Part model, mm, in its own coordinate system. Face numbers are marked on the shaded views. A direction names the side the tool comes from. Coordinates: 2 decimals unless noted, no trailing zeros. Loops run counter-clockwise (first coordinate to the right, second up) from the corner with the lowest first, then second, coordinate; pieces in that order, holes last. Notation, with made-up numbers: (87, 27.25) -> (114, 27.25) arc R22 ccw to (114, 38.25) -> close; hole circle Ø7 at (-8.5, 3). An arc over 180 degrees is marked (long way). Use one line per item in the form item = value. Start each with the question number.
(1) Band-saw the part on C-C on y = 3. Give the cut face in (x, z).
(2) Drill centre lines: L1, parallel to X at y = 0, z = 21; L2, parallel to Y at x = 4.5, z = 21.75; L3, parallel to Z at x = 0, y = -1.75. Where is each one in solid material? Low to high. Write a range as [from, to].
(3) Pin check, flat tips, straight feed: P1, Ø1.8, axis at x = -4.5, y = 0, coming from the +Z side; P2, Ø5, axis at x = 1.5, y = 1, coming from the -Z side; P3, Ø1.3, axis at x = -4.5, y = -3.5, coming from the -Z side; P4, Ø1.8, axis at x = -0.5, z = 27, coming from the +Y side. Stop position of each tip, or through.
(4) Band-saw the part on B-B on z = 4.5. Give the cut face in (x, y), then the cut area to 3 significant figures.
(5) 3-axis set-ups, long thin cutter, end or side, ignore diameter. For the marked faces 1, 2, 3, 4 and 5: which of +Z, -Z, +X, -X, +Y, -Y reach the whole face in a straight line?
(6) Band-saw the part on A-A on z = 23. Give the cut face in (x, y), then the cut area to 3 significant figures.
(7) Band-saw the part on D-D on z = 29.5. Give the cut face in (x, y).
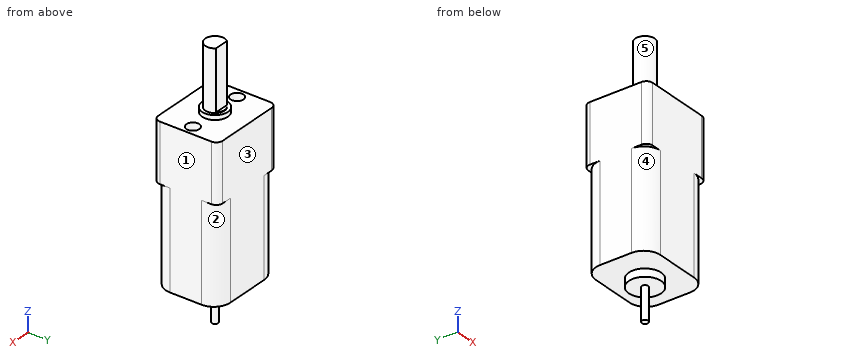
```python
from build123d import *

# Parameters (mm, degrees)
BOSS_EXTRUDE1_DEPTH        = 15
BOSS_EXTRUDE2_DEPTH        = 9
SKETCH3_R                  = 2
BOSS_EXTRUDE3_DEPTH        = 0.7
SKETCH4_R                  = 1.5
BOSS_EXTRUDE4_DEPTH        = 9.3
SKETCH5_W                  = 3
SKETCH5_H                  = 1
CUT_EXTRUDE1_DEPTH         = 9.2
SKETCH6_R                  = 2.5
BOSS_EXTRUDE5_DEPTH        = 1.2
SKETCH7_R                  = 0.5
BOSS_EXTRUDE6_DEPTH        = 5
M1_6_CLEARANCE_HOLE1_D     = 2
M1_6_CLEARANCE_HOLE1_DEPTH = 7
M1_6_CLEARANCE_HOLE1_TIP   = 0.600860619


with BuildPart() as part:
    # Sketch1 → Boss-Extrude1 (new body)
    with BuildSketch(Plane.XY):
        with BuildLine():
            Line((3.45, -5), (-3.45, -5))
            ThreePointArc((-3.45, -5), (-5.253122292, -4.253122292), (-6, -2.45))
            Line((-6, -2.45), (-6, 2.45))
            ThreePointArc((-6, 2.45), (-5.253122292, 4.253122292), (-3.45, 5))
            Line((-3.45, 5), (3.45, 5))
            ThreePointArc((3.45, 5), (5.253122292, 4.253122292), (6, 2.45))
            Line((6, 2.45), (6, -2.45))
            ThreePointArc((6, -2.45), (5.253122292, -4.253122292), (3.45, -5))
        make_face()
    extrude(amount=BOSS_EXTRUDE1_DEPTH)

    # Sketch2 → Boss-Extrude2 (add)
    with BuildSketch(Plane.XY.offset(15)):
        with BuildLine():
            Line((5, -5), (-5, -5))
            ThreePointArc((-5, -5), (-5.707106781, -4.707106781), (-6, -4))
            Line((-6, -4), (-6, 4))
            ThreePointArc((-6, 4), (-5.707106781, 4.707106781), (-5, 5))
            Line((-5, 5), (5, 5))
            ThreePointArc((5, 5), (5.707106781, 4.707106781), (6, 4))
            Line((6, 4), (6, -4))
            ThreePointArc((6, -4), (5.707106781, -4.707106781), (5, -5))
        make_face()
    extrude(amount=BOSS_EXTRUDE2_DEPTH)

    # Sketch3 → Boss-Extrude3 (add)
    with BuildSketch(Plane.XY.offset(24)):
        Circle(SKETCH3_R)
    extrude(amount=BOSS_EXTRUDE3_DEPTH)

    # Sketch4 → Boss-Extrude4 (add)
    with BuildSketch(Plane.XY.offset(24.7)):
        Circle(SKETCH4_R)
    extrude(amount=BOSS_EXTRUDE4_DEPTH)

    # Sketch5 → Cut-Extrude1 (cut)
    with BuildSketch(Plane.XY.offset(34)):
        with Locations((0, 1.5)):
            Rectangle(SKETCH5_W, SKETCH5_H)
    extrude(amount=-CUT_EXTRUDE1_DEPTH, mode=Mode.SUBTRACT)

    # Sketch6 → Boss-Extrude5 (add)
    with BuildSketch(Plane(origin=(0, 0, 0), x_dir=(-1, 0, 0), z_dir=(0, 0, -1))):
        Circle(SKETCH6_R)
    extrude(amount=BOSS_EXTRUDE5_DEPTH)

    # Sketch7 → Boss-Extrude6 (add)
    with BuildSketch(Plane(origin=(0, 0, -1.2), x_dir=(-1, 0, 0), z_dir=(0, 0, -1))):
        Circle(SKETCH7_R)
    extrude(amount=BOSS_EXTRUDE6_DEPTH)

    # M1.6 Clearance Hole1
    with Locations(Plane.XY.offset(24)):
        with Locations((-4.5, 0), (4.5, 0)):
            Hole(M1_6_CLEARANCE_HOLE1_D / 2, depth=M1_6_CLEARANCE_HOLE1_DEPTH)
            with Locations((0, 0, -(M1_6_CLEARANCE_HOLE1_DEPTH + M1_6_CLEARANCE_HOLE1_TIP / 2))):  # 118° drill point
                Cone(0, M1_6_CLEARANCE_HOLE1_D / 2, M1_6_CLEARANCE_HOLE1_TIP, mode=Mode.SUBTRACT)


solid = part.part
```
A:
q1.outline = (-6, 15) -> (-5.94, 15) -> (-5.94, 0) -> (5.94, 0) -> (5.94, 15) -> (6, 15) -> (6, 24) -> (-6, 24) -> close
q2.L1 = [-6, -5.5], [-3.5, 3.5], [5.5, 6]
q2.L2 = [-5, -1], [1, 5]
q2.L3 = [-1.2, 24.7]
q3.P1 = 16.94
q3.P2 = -6.2
q3.P3 = 0
q3.P4 = 1
q4.outline = (-6, -2.45) arc R2.55 ccw to (-3.45, -5) -> (3.45, -5) arc R2.55 ccw to (6, -2.45) -> (6, 2.45) arc R2.55 ccw to (3.45, 5) -> (-3.45, 5) arc R2.55 ccw to (-6, 2.45) -> close
q4.area = 114 mm²
q5.face_1 = +Z, -Z, +X, +Y, -Y
q5.face_2 = -Z, +X, +Y
q5.face_3 = +Z, -Z, +X, -X, +Y
q5.face_4 = -Z, -X, -Y
q5.face_5 = +Z
q6.outline = (-6, -4) arc R1 ccw to (-5, -5) -> (5, -5) arc R1 ccw to (6, -4) -> (6, 4) arc R1 ccw to (5, 5) -> (-5, 5) arc R1 ccw to (-6, 4) -> close; hole circle Ø2 at (-4.5, 0); hole circle Ø2 at (4.5, 0)
q6.area = 113 mm²
q7.outline = (-1.12, 1) arc R1.5 ccw (long way) to (1.12, 1) -> close
